from build123d import *

# Parameters (mm, degrees)
F0_W      = 40
F0_H      = 32
F1_DEPTH  = 105
F2_R      = 7.5
F3_DEPTH  = 75
F4_R      = 3
F5_DEPTH  = 105.001
F7_R      = 67.5
F8_DEPTH  = 6
F10_R     = 3
F11_DEPTH = 15


with BuildPart() as f1:
    # F0 (on Front) → F1 (new body)
    with BuildSketch(Plane.XZ):
        with Locations((-20, 16)):
            Rectangle(F0_W, F0_H)
    extrude(amount=-F1_DEPTH)

    # F2 (on face) → F3 (cut)
    with BuildSketch(Plane.XZ):
        with Locations((-20, 16)):
            Circle(F2_R)
    extrude(amount=-F3_DEPTH, mode=Mode.SUBTRACT)

    # F4 (on Front) → F5 (cut, through all)
    with BuildSketch(Plane.XZ):
        with Locations((-20, 11.5)):
            Circle(F4_R)
    extrude(amount=-F5_DEPTH, mode=Mode.SUBTRACT)

    # F7 (on offset) → F8 (cut)
    with BuildSketch(Plane.XZ.offset(-20)):
        with Locations((-20, 96.5)):
            Circle(F7_R)
    extrude(amount=-F8_DEPTH, mode=Mode.SUBTRACT)

    # F10 (on offset) → F11 (cut)
    with BuildSketch(Plane.XY.offset(32)):
        with Locations((-8, 23)):
            Circle(F10_R)
    extrude(amount=-F11_DEPTH, mode=Mode.SUBTRACT)


solid = f1.part
Work out the finished part from the listing and answer in its coordinate system (mm). A direction names the side the tool comes from. Give positions to 0.01 mm unless a question says otherwise; leave off trailing zeros. Loops run counter-clockwise (first coordinate to the right, second up) from the corner with the lowest first, then second, coordinate; pieces in that order, holes last. Notation, with made-up numbers: (-6.75, 81.5) - (49.25, 81.5) arc R31 ccw to (49.25, 110.5) - close; hole circle Ø2 at (14, 50). An arc over 180 degrees is marked (long way). Answer in a Markdown table with one row per item. Add a question column.
Q1. The part is cut by section D-D (x = -6). Determine the outline of the cut face in (y, z).
Q2. The part is cut by section A-A (z = 10.5). Determine the outline of the cut face in (x, y).
Q3. Determine the mould class of faces 4 (the cylindrical face through (-25.5, 37, 21.1)), 5 (the flat face through (-20, 26, 31)), 6 (the flat face through (-16, 0, 9)) for opening direction Y: released by +Y, released by -Y, zero draft, split by the parting line, or undercut.
Q4. The part is cut by section B-B (y = 39). Determine the outline of the cut face in (x, z), and give its area (3 significant figures).
Q5. A tool of negligible diameter and unlimited length cuts with its end or side. For faces 1 (the flat face through (-8, 23, 17)), 2 (the flat face through (-40, 52, 16)), 3 (the flat face through (-20, 75, 16)), from which of +Z, -Z, +X, -X, +Y, -Y can it reach the whole face along a straight path? Write none if from no direction.
Q6. The part is cut by section C-C (z = 16). Determine the outline of the cut face in (x, y), and give its area (4 significant figures).
Q7. Consider line 1 along Y through (x, z) = (-11, 30); line 2 along X through (y, z) = (46.5, 16); line 3 along Z through (x, y) = (-20, 46). Determine where each line is inside the solid, lowest interval first.
Q8. Each of these flat-tipped pins is pushed along its axis until it touches: P1, Ø8, axis at x = -19.5, z = 18, coming from the -Y side; P2, Ø1.8, axis at x = -7, y = 23, coming from the +Z side; P3, Ø3.5, axis at x = -20, z = 11.5, coming from the -Y side. Where does it stop, or does it pass through?
Solution:
| question | item | result |
|---|---|---|
| 1 | outline | (0, 0) - (105, 0) - (105, 32) - (26, 32) - (26, 30.47) - (25.24, 30.47) - (25.24, 17) - (20.76, 17) - (20.76, 30.47) - (20, 30.47) - (20, 32) - (0, 32) - close |
| 2 | outline | (-40, 0) - (-25.1, 0) - (-25.1, 75) - (-22.83, 75) - (-22.83, 105) - (-40, 105) - close; (-17.17, 75) - (-14.9, 75) - (-14.9, 0) - (0, 0) - (0, 105) - (-17.17, 105) - close |
| 3 | face 4 | zero draft |
| 3 | face 5 | undercut |
| 3 | face 6 | released by -Y |
| 4 | outline | (-40, 0) - (0, 0) - (0, 32) - (-40, 32) - close; hole circle Ø15 at (-20, 16) |
| 4 | area | 1,100 mm² |
| 5 | face 1 | +Z |
| 5 | face 2 | +Z, -Z, -X, +Y, -Y |
| 5 | face 3 | -Y |
| 6 | outline | (-40, 0) - (-27.5, 0) - (-27.5, 75) - (-12.5, 75) - (-12.5, 0) - (0, 0) - (0, 105) - (-40, 105) - close |
| 6 | area | 3,075 mm² |
| 7 | line 1 | y = 0 to 20, 26 to 105 |
| 7 | line 2 | x = -40 to -27.5, -12.5 to 0 |
| 7 | line 3 | z = 0 to 8.5, 23.5 to 32 |
| 8 | P1 | stops at y = 75 |
| 8 | P2 | stops at z = 17 |
| 8 | P3 | passes through |
